from build123d import *

# Parameters (mm, degrees)
F0_W       = 19.05
F0_H       = 19.05
F0_W_2     = 15.875
F0_H_2     = 15.875
F1_DEPTH   = 196.85
F2_R       = 2.15265
F1_FACE1_W = 19.05
F1_FACE1_H = 393.7
F3_DEPTH   = 25.4


with BuildPart() as f1:
    # F0 (on Front) → F1 (new body, symmetric)
    with BuildSketch(Plane.XZ):
        Rectangle(F0_W, F0_H)
        Rectangle(F0_W_2, F0_H_2, mode=Mode.SUBTRACT)
    extrude(amount=F1_DEPTH, both=True)

    # F2 (on face) + F1_face1 (on face) → F3 (cut)
    with BuildSketch(Plane.XY.offset(9.525)):
        with Locations((0, 12.7)):
            Circle(F2_R)
        with Locations((0, -12.7)):
            Circle(F2_R)
        with Locations((0, 76.2)):
            Circle(F2_R)
        with Locations((0, 50.8)):
            Circle(F2_R)
        with Locations((0, 139.7)):
            Circle(F2_R)
        with Locations((0, 114.3)):
            Circle(F2_R)
        with Locations((0, -50.8)):
            Circle(F2_R)
        with Locations((0, -76.2)):
            Circle(F2_R)
        with Locations((0, -114.3)):
            Circle(F2_R)
        with Locations((0, -139.7)):
            Circle(F2_R)
    with BuildSketch(Plane(origin=(0, 0, -9.525), x_dir=(1, 0, 0), z_dir=(0, 0, -1))):
        Rectangle(F1_FACE1_W, F1_FACE1_H)
    extrude(amount=-F3_DEPTH, dir=(0, 0, 1), mode=Mode.SUBTRACT)


solid = f1.part
The listing builds one solid part. Answer for the finished solid, in the listing's coordinates (mm). A direction names the side the tool comes from. Coordinates: 2 decimals unless noted, no trailing zeros. Order: outer loops, then holes, each group sorted by start corner. A loop starts at its lowest first (then second) coordinate and runs counter-clockwise, first axis right, second up.
Q1. Given P1, Ø7, axis at x = 0, y = 76.2, coming from the -Z side (3 decimals), flat-ended and moving along its own axis, determine where the tip first touches the part or whether it passes through.
Q2. Consider line 1 (Z direction, x = 3.75, y = 41) (1 decimal); line 2 (X direction, y = 139.7, z = -9.05) (3 decimals). Determine where each line is inside the solid, lowest interval first.
Q3. For a pull along X with two mould halves and no side action, classify faces 3 (the face through (0, -3, 7.938)), 4 (the face through (7.938, -3, 0)), 5 (the face through (-9.525, -3, 0)), 6 (the face through (-9, -196.85, 0)) as pulls with the +X half, pulls with the -X half, needs draft (parallel to the pull), parting line crosses it, or undercut.
Q4. Which of the six approach directions +Z, -Z, +X, -X, +Y, -Y give full straight-line access (tool end or side, diameter ignored) to faces 1 (the face through (-7.938, -3, 0)), 2 (the face through (9.525, -3, 0))?
Q5. A cutting plane is placed at B-B, the plane y = -89. Write down the section's boundary in (x, z) (1 decimal).
Answers follow:
1. P1: stops at z = -9.525
2. line 1: z = -9.5 to -7.9, 7.9 to 9.5
2. line 2: x = -9.525 to -2.153, 2.153 to 9.525
3. face 3: undercut
3. face 4: undercut
3. face 5: pulls with the -X half
3. face 6: needs draft
4. face 1: +Y, -Y
4. face 2: +Z, -Z, +X, +Y, -Y
5. outline: (-9.5, -9.5) - (9.5, -9.5) - (9.5, 9.5) - (-9.5, 9.5) - close; hole (-7.9, -7.9) - (7.9, -7.9) - (7.9, 7.9) - (-7.9, 7.9) - close
